```python
from build123d import *

# Parameters (mm, degrees)
F1_DEPTH = 6
F2_R     = 3
F3_DEPTH = 2


with BuildPart() as f1:
    # F0 (on Front) → F1 (new body)
    with BuildSketch(Plane.XZ):
        with BuildLine():
            Line((-42.0022320835, 24.25), (-2.3, 1.3279056191))
            Line((-2.3, 1.3279056191), (-2.3, 3.9837168574))
            Line((-2.3, 3.9837168574), (-24.25, 42.0022320835))
            ThreePointArc((-24.25, 42.0022320835), (-25.3773506768, 41.8495104065), (-26.2876419557, 42.5318689974))
            ThreePointArc((-26.2876419557, 42.5318689974), (-35.3553390593, 35.3553390593), (-42.5318689974, 26.2876419557))
            ThreePointArc((-42.5318689974, 26.2876419557), (-41.9966434633, 25.7402358449), (-41.8012701892, 25))
            ThreePointArc((-41.8012701892, 25), (-41.8523814498, 24.6117714323), (-42.0022320835, 24.25))
        make_face()
        with BuildLine():
            Line((-2.3, 30), (0, 30))
            Line((0, 30), (0, 48.5))
            ThreePointArc((0, 48.5), (-1.0526751636, 48.9314144863), (-1.4998312405, 49.9775))
            ThreePointArc((-1.4998312405, 49.9775), (-12.9409522551, 48.2962913145), (-23.6898580443, 44.0317002379))
            ThreePointArc((-23.6898580443, 44.0317002379), (-23.5482402173, 43.678620866), (-23.5, 43.3012701892))
            ThreePointArc((-23.5, 43.3012701892), (-23.7009618943, 42.5512701892), (-24.25, 42.0022320835))
            Line((-24.25, 42.0022320835), (-2.3, 3.9837168574))
            Line((-2.3, 3.9837168574), (-2.3, 30))
        make_face()
        with BuildLine():
            Line((0, 48.5), (0, 30))
            Line((0, 30), (2.3, 30))
            Line((2.3, 30), (2.3, 3.9837168574))
            Line((2.3, 3.9837168574), (24.25, 42.0022320835))
            ThreePointArc((24.25, 42.0022320835), (23.5540638096, 42.9021855701), (23.6898580443, 44.0317002379))
            ThreePointArc((23.6898580443, 44.0317002379), (12.9409522551, 48.2962913145), (1.4998312405, 49.9775))
            ThreePointArc((1.4998312405, 49.9775), (1.0526751636, 48.9314144863), (0, 48.5))
        make_face()
        with BuildLine():
            Line((2.3, 1.3279056191), (42.0022320835, 24.25))
            ThreePointArc((42.0022320835, 24.25), (41.8495104065, 25.3773506768), (42.5318689974, 26.2876419557))
            ThreePointArc((42.5318689974, 26.2876419557), (35.3553390593, 35.3553390593), (26.2876419557, 42.5318689974))
            ThreePointArc((26.2876419557, 42.5318689974), (25.3773506768, 41.8495104065), (24.25, 42.0022320835))
            Line((24.25, 42.0022320835), (2.3, 3.9837168574))
            Line((2.3, 3.9837168574), (2.3, 1.3279056191))
        make_face()
        with BuildLine():
            ThreePointArc((48.5, 0), (48.9314144863, 1.0526751636), (49.9775, 1.4998312405))
            ThreePointArc((49.9775, 1.4998312405), (48.2962913145, 12.9409522551), (44.0317002379, 23.6898580443))
            ThreePointArc((44.0317002379, 23.6898580443), (42.9021855701, 23.5540638096), (42.0022320835, 24.25))
            Line((42.0022320835, 24.25), (2.3, 1.3279056191))
            Line((2.3, 1.3279056191), (2.3, 0))
            Line((2.3, 0), (48.5, 0))
        make_face()
        with BuildLine():
            ThreePointArc((44.0317002379, -23.6898580443), (48.2962913145, -12.9409522551), (49.9775, -1.4998312405))
            ThreePointArc((49.9775, -1.4998312405), (48.9314144863, -1.0526751636), (48.5, 0))
            Line((48.5, 0), (2.3, 0))
            Line((2.3, 0), (0, 0))
            Line((0, 0), (42.0022320835, -24.25))
            ThreePointArc((42.0022320835, -24.25), (42.9021855701, -23.5540638096), (44.0317002379, -23.6898580443))
        make_face()
        with BuildLine():
            ThreePointArc((42.5318689974, -26.2876419557), (41.8495104065, -25.3773506768), (42.0022320835, -24.25))
            Line((42.0022320835, -24.25), (0, 0))
            Line((0, 0), (24.25, -42.0022320835))
            ThreePointArc((24.25, -42.0022320835), (25.3773506768, -41.8495104065), (26.2876419557, -42.5318689974))
            ThreePointArc((26.2876419557, -42.5318689974), (35.3553390593, -35.3553390593), (42.5318689974, -26.2876419557))
        make_face()
        with BuildLine():
            Line((24.25, -42.0022320835), (0, 0))
            Line((0, 0), (0, -48.5))
            ThreePointArc((0, -48.5), (1.0526751636, -48.9314144863), (1.4998312405, -49.9775))
            ThreePointArc((1.4998312405, -49.9775), (12.9409522551, -48.2962913145), (23.6898580443, -44.0317002379))
            ThreePointArc((23.6898580443, -44.0317002379), (23.5540638096, -42.9021855701), (24.25, -42.0022320835))
        make_face()
        with BuildLine():
            Line((0, -48.5), (0, 0))
            Line((0, 0), (-24.25, -42.0022320835))
            ThreePointArc((-24.25, -42.0022320835), (-23.7009618943, -42.5512701892), (-23.5, -43.3012701892))
            ThreePointArc((-23.5, -43.3012701892), (-23.5482402173, -43.678620866), (-23.6898580443, -44.0317002379))
            ThreePointArc((-23.6898580443, -44.0317002379), (-12.9409522551, -48.2962913145), (-1.4998312405, -49.9775))
            ThreePointArc((-1.4998312405, -49.9775), (-1.0526751636, -48.9314144863), (0, -48.5))
        make_face()
        with BuildLine():
            Line((-24.25, -42.0022320835), (0, 0))
            Line((0, 0), (-42.0022320835, -24.25))
            ThreePointArc((-42.0022320835, -24.25), (-41.8523814498, -24.6117714323), (-41.8012701892, -25))
            ThreePointArc((-41.8012701892, -25), (-41.9966434633, -25.7402358449), (-42.5318689974, -26.2876419557))
            ThreePointArc((-42.5318689974, -26.2876419557), (-35.3553390593, -35.3553390593), (-26.2876419557, -42.5318689974))
            ThreePointArc((-26.2876419557, -42.5318689974), (-25.3773506768, -41.8495104065), (-24.25, -42.0022320835))
        make_face()
        with BuildLine():
            Line((-42.0022320835, -24.25), (0, 0))
            Line((0, 0), (-2.3, 0))
            Line((-2.3, 0), (-48.5, 0))
            ThreePointArc((-48.5, 0), (-48.9314144863, -1.0526751636), (-49.9775, -1.4998312405))
            ThreePointArc((-49.9775, -1.4998312405), (-48.2962913145, -12.9409522551), (-44.0317002379, -23.6898580443))
            ThreePointArc((-44.0317002379, -23.6898580443), (-42.9021855701, -23.5540638096), (-42.0022320835, -24.25))
        make_face()
        with BuildLine():
            Line((-48.5, 0), (-2.3, 0))
            Line((-2.3, 0), (-2.3, 1.3279056191))
            Line((-2.3, 1.3279056191), (-42.0022320835, 24.25))
            ThreePointArc((-42.0022320835, 24.25), (-42.9021855701, 23.5540638096), (-44.0317002379, 23.6898580443))
            ThreePointArc((-44.0317002379, 23.6898580443), (-48.2962913145, 12.9409522551), (-49.9775, 1.4998312405))
            ThreePointArc((-49.9775, 1.4998312405), (-48.9314144863, 1.0526751636), (-48.5, 0))
        make_face()
    extrude(amount=F1_DEPTH)

    # F2 (on face) → F3 (join)
    with BuildSketch(Plane.XZ.offset(6)):
        with BuildLine():
            ThreePointArc((3, 42.5), (2.1213203436, 44.6213203436), (0, 45.5))
            ThreePointArc((0, 45.5), (-2.1213203436, 40.3786796564), (3, 42.5))
        make_face()
        with BuildLine():
            ThreePointArc((24.25, 36.8060796608), (23.8480762114, 38.3060796608), (22.75, 39.4041558722))
            ThreePointArc((22.75, 39.4041558722), (18.6519237886, 35.3060796608), (24.25, 36.8060796608))
        make_face()
        with BuildLine():
            ThreePointArc((39.8060796608, 21.25), (39.7038571397, 22.0264571353), (39.4041558722, 22.75))
            ThreePointArc((39.4041558722, 22.75), (33.908302182, 20.4735428647), (39.8060796608, 21.25))
        make_face()
        with Locations((42.5, 0)):
            Circle(F2_R)
        with BuildLine():
            ThreePointArc((39.8060796608, -21.25), (33.908302182, -20.4735428647), (39.4041558722, -22.75))
            ThreePointArc((39.4041558722, -22.75), (39.7038571397, -22.0264571353), (39.8060796608, -21.25))
        make_face()
        with BuildLine():
            ThreePointArc((24.25, -36.8060796608), (18.6519237886, -35.3060796608), (22.75, -39.4041558722))
            ThreePointArc((22.75, -39.4041558722), (23.8480762114, -38.3060796608), (24.25, -36.8060796608))
        make_face()
        with BuildLine():
            ThreePointArc((3, -42.5), (-2.1213203436, -40.3786796564), (0, -45.5))
            ThreePointArc((0, -45.5), (2.1213203436, -44.6213203436), (3, -42.5))
        make_face()
        with BuildLine():
            ThreePointArc((-18.25, -36.8060796608), (-22.75, -34.2080034495), (-22.75, -39.4041558722))
            ThreePointArc((-22.75, -39.4041558722), (-19.75, -39.4041558722), (-18.25, -36.8060796608))
        make_face()
        with BuildLine():
            ThreePointArc((-33.8060796608, -21.25), (-37.5825367961, -18.3522225211), (-39.4041558722, -22.75))
            ThreePointArc((-39.4041558722, -22.75), (-36.0296225255, -24.1477774789), (-33.8060796608, -21.25))
        make_face()
        with BuildLine():
            ThreePointArc((-39.5, 0), (-42.5, 3), (-45.5, 0))
            ThreePointArc((-45.5, 0), (-42.5, -3), (-39.5, 0))
        make_face()
        with BuildLine():
            ThreePointArc((-33.8060796608, 21.25), (-36.0296225255, 24.1477774789), (-39.4041558722, 22.75))
            ThreePointArc((-39.4041558722, 22.75), (-37.5825367961, 18.3522225211), (-33.8060796608, 21.25))
        make_face()
        with BuildLine():
            ThreePointArc((-18.25, 36.8060796608), (-19.75, 39.4041558722), (-22.75, 39.4041558722))
            ThreePointArc((-22.75, 39.4041558722), (-22.75, 34.2080034495), (-18.25, 36.8060796608))
        make_face()
    extrude(amount=F3_DEPTH)


solid = f1.part
```
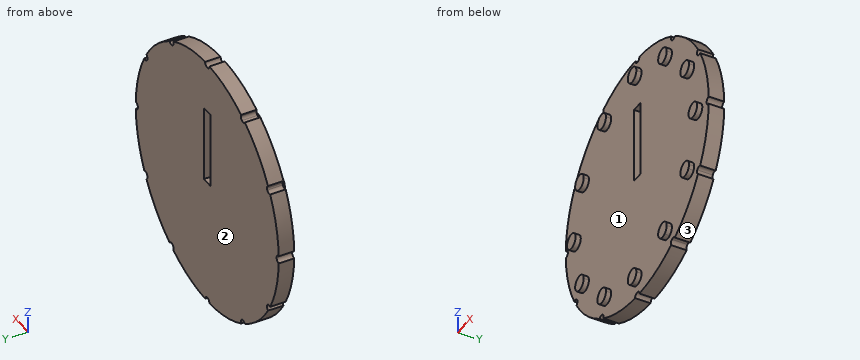
The model under review builds one solid part; all positions refer to its coordinate system, in mm. Face numbers are marked on the shaded views. Give positions to 0.01 mm unless a question says otherwise; leave off trailing zeros. Write each loop counter-clockwise with the first axis right and the second up, starting at its lowest first coordinate (ties: lowest second). Pieces come first, ordered by that corner, then holes.
(1) For P1, Ø3, axis at y = -1.5, z = 7.5, coming from the -X side; P2, Ø3, axis at x = 39.5, z = -10, coming from the -Y side; P3, Ø3, axis at y = -3.5, z = 20.5, coming from the +X side, all flat-tipped, find the tip position at first contact; note any pin that passes through.
(2) Consider section C-C, the plane z = -28.5. Give the boundary of the cut face in (x, y), and give its area (3 significant figures).
(3) Consider section D-D, the plane x = 12.5. Give the boundary of the cut face in (y, z).
(4) The part is to be moulded in two halves that separate along X. For the marked faces 1, 2 and 3, say which applies: released by +X, released by -X, zero draft, split by the parting line, or undercut.
(5) Consider section B-B, the plane x = -35.5. Give the boundary of the cut face in (y, z).
(6) Consider section A-A, the plane z = 13. Give the boundary of the cut face in (x, y), and give its area (3 significant figures).
(7) To check wall thickness, follow L1, parallel to Y at x = 22, z = 16; L2, parallel to X at y = -4.5, z = 15; L3, parallel to Z at x = -14.5, y = -4.75. State the ranges of each line that lie inside material, in increasing order.
Returned:
1. P1: stops at x = -49.64
1. P2: stops at y = -6
1. P3: stops at x = 46.25
2. outline: (-41.08, -6) - (41.08, -6) - (41.08, 0) - (-41.08, 0) - close
2. area: 493 mm2
3. outline: (-6, -48.41) - (0, -48.41) - (0, 48.41) - (-6, 48.41) - close
4. face 1: undercut
4. face 2: zero draft
4. face 3: released by +X
5. outline: (-8, -23.95) - (-6, -23.95) - (-6, -35.21) - (0, -35.21) - (0, 35.21) - (-6, 35.21) - (-6, 23.95) - (-8, 23.95) - (-8, 18.55) - (-6, 18.55) - (-6, -18.55) - (-8, -18.55) - close
6. outline: (-48.28, -6) - (-2.3, -6) - (-2.3, 0) - (-48.28, 0) - close; (2.3, -6) - (48.28, -6) - (48.28, 0) - (2.3, 0) - close
6. area: 552 mm2
7. L1: y = -6 to 0
7. L2: x = -47.7 to -2.3, 2.3 to 47.7
7. L3: z = -47.85 to 47.85
